from build123d import *

# Parameters (mm, degrees)
F0_W     = 150
F0_H     = 140
F1_DEPTH = 85
F2_R     = 11.08773
F3_DEPTH = 25
F4_R     = 60
F5_DEPTH = 10


with BuildPart() as f1:
    # F0 (on Top) → F1 (new body)
    with BuildSketch(Plane.XY):
        Rectangle(F0_W, F0_H)
    extrude(amount=F1_DEPTH)

    # F2 (on face) → F3 (cut)
    with BuildSketch(Plane.XZ.offset(70)):
        with Locations((-63.034661, 44.377975)):
            Circle(F2_R)
    extrude(amount=-F3_DEPTH, mode=Mode.SUBTRACT)

    # F4 (on face) → F5 (cut)
    with BuildSketch(Plane.XY.offset(85)):
        with Locations((10, 0)):
            Circle(F4_R)
    extrude(amount=-F5_DEPTH, mode=Mode.SUBTRACT)


solid = f1.part
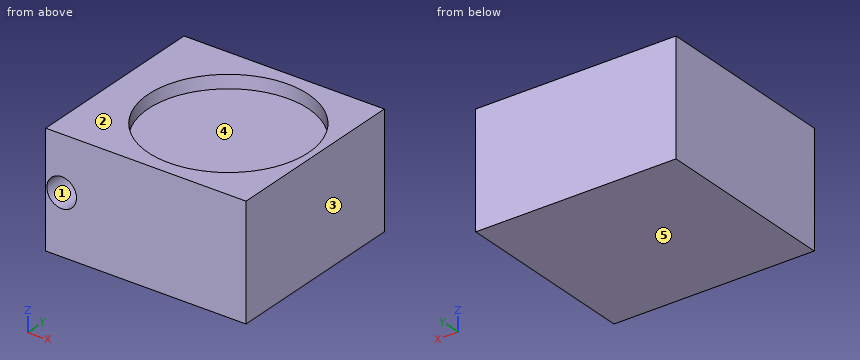
Read the model definition and answer for the solid it produces. Units are mm, in the model's axes. Face numbers are marked on the shaded views. A direction names the side the tool comes from. Give positions to 0.01 mm unless a question says otherwise; leave off trailing zeros. Write each loop counter-clockwise with the first axis right and the second up, starting at its lowest first coordinate (ties: lowest second). Pieces come first, ordered by that corner, then holes. Notation, with made-up numbers: (73.5, 67) -> (96.5, 67) arc R9 ccw to (96.5, 83) -> close; hole circle Ø9 at (89.25, 84). An arc over 180 degrees is marked (long way). Answer as a JSON object with one key per item and string values. Group by question number.
1) The mould has two halves that part along Z. Classify the marked faces 1, 2 and 3: +Z half, -Z half, draft (parallel to the pull), parting line (faces both ways), or undercut.
2) A tool of negligible diameter and unlimited length cuts with its end or side. For the marked faces 4 and 5, from which of +Z, -Z, +X, -X, +Y, -Y can it reach the whole face along a straight path? Write none if from no direction.
3) Each of these flat-tipped pins is pushed along its axis until it touches: P1, Ø6, axis at x = -14, y = -4, coming from the +Z side; P2, Ø6.5, axis at x = -62, z = 43, coming from the -Y side. Where does it stop, or does it pass through?
4) Find section B-B (y = 0). Write down the section's boundary in (x, z).
5) Consider L1, parallel to Y at x = 10, z = 77; L2, parallel to Z at x = 52, y = 2; L3, parallel to Y at x = 36, z = 80. Determine where each line is inside the solid, lowest interval first. Write a range as from..to.
6) Find section A-A (x = 10). Write down the section's boundary in (y, z), and give its area (3 significant figures).
7) Find section C-C (y = -56.5). Write down the section's boundary in (x, z), and give its area (3 significant figures).
Values follow:
{
 "1": {"face 1": "undercut", "face 2": "+Z half", "face 3": "draft"},
 "2": {"face 4": "+Z", "face 5": "-Z, +X, -X, +Y, -Y"},
 "3": {"P1": "stops at z = 75", "P2": "stops at y = -45"},
 "4": {"outline": "(-75, 0) -> (75, 0) -> (75, 85) -> (70, 85) -> (70, 75) -> (-50, 75) -> (-50, 85) -> (-75, 85) -> close"},
 "5": {"L1": "y = -70..-60, 60..70", "L2": "z = 0..75", "L3": "y = -70..-54.07, 54.07..70"},
 "6": {"outline": "(-70, 0) -> (70, 0) -> (70, 85) -> (60, 85) -> (60, 75) -> (-60, 75) -> (-60, 85) -> (-70, 85) -> close", "area": "10,700 mm2"},
 "7": {"outline": "(-75, 0) -> (75, 0) -> (75, 85) -> (30.19, 85) -> (30.19, 75) -> (-10.19, 75) -> (-10.19, 85) -> (-75, 85) -> close; hole circle Ø22.18 at (-63.03, 44.38)", "area": "12,000 mm2"}
}
